```python
from build123d import *

# Parameters (mm, degrees)
SKETCH1_R = 20
SKETCH2_R = 16
SKETCH3_R = 17
SKETCH4_R = 10


with BuildPart() as part:
    # Sketch1 → Loft1 section 0
    with BuildSketch(Plane.XY):
        Circle(SKETCH1_R)
    # Sketch2 → Loft1 section 1
    with BuildSketch(Plane.XY.offset(100)):
        Circle(SKETCH2_R)
    loft()

    # Sketch3 → section 1 of loft4
    with BuildSketch(Plane.XY.offset(200), mode=Mode.PRIVATE) as loft4_s1:
        Circle(SKETCH3_R)
    # loft up to a face of the part (loft4)
    loft([Face(Wire([part.edges().sort_by_distance((-10.952753695, 11.663498039, 100))[0]])), loft4_s1.sketch])

    # Sketch4 → section 1 of loft5
    with BuildSketch(Plane.XY.offset(300), mode=Mode.PRIVATE) as loft5_s1:
        Circle(SKETCH4_R)
    # loft up to a face of the part (loft5)
    loft([Face(Wire([part.edges().sort_by_distance((-11.637300801, 12.392466666, 200))[0]])), loft5_s1.sketch])


solid = part.part
```
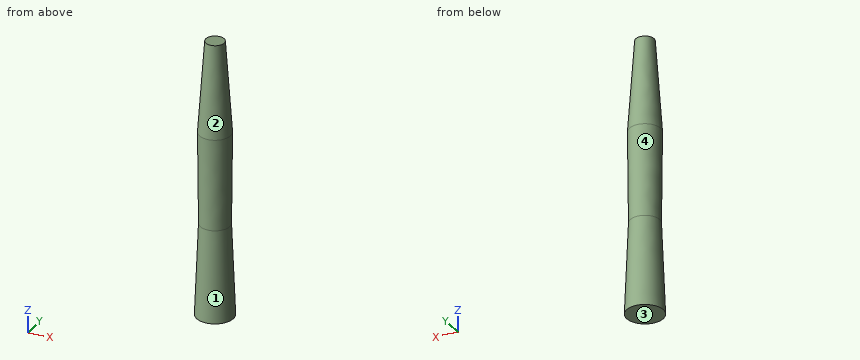
Read the model definition and answer for the solid it produces. Units are mm, in the model's axes. Face numbers are marked on the shaded views. Give positions to 0.01 mm unless a question says otherwise; leave off trailing zeros. Order: outer loops, then holes, each group sorted by start corner. A loop starts at its lowest first (then second) coordinate and runs counter-clockwise, first axis right, second up. Notation, with made-up numbers: (65, 36.25) -> (82, 36.25) arc R21 ccw to (82, 49.25) -> close; hole circle Ø10 at (25, 14.5). An arc over 180 degrees is marked (long way). Write item = value, one per line.
1. Given pin 1 (10 mm diameter, centred on y = -2, z = 189.5, fed in from -X); pin 2 (10 mm diameter, centred on x = 11, y = -15.5, fed in from -Z); pin 3 (8 mm diameter, centred on x = 15.5, z = 36.5, fed in from -Y); pin 4 (2 mm diameter, centred on y = 15, z = 246, fed in from +X) (3 decimals), each flat-ended and moving along its own axis, determine where each tip first touches the part or whether it passes through.
Numbers:
pin_1 = -16.94
pin_2 = 0
pin_3 = -14.55
pin_4 = through
2. A cutting plane is placed at B-B, the plane z = 205. Write down the section's boundary in (x, y), and give its area (3 significant figures).
Numbers:
outline = circle Ø33.3 at (0, 0)
area = 871 mm²
3. The mould has two halves that part along Z. Classify the marked faces 1, 2, 3 and 4: +Z half, -Z half, draft (parallel to the pull), parting line (faces both ways), or undercut.
Numbers:
face_1 = undercut
face_2 = +Z half
face_3 = -Z half
face_4 = undercut
4. A cutting plane is placed at A-A, the plane z = 26. Write down the section's boundary in (x, y), and give its area (3 significant figures).
Numbers:
outline = circle Ø37.92 at (0, 0)
area = 1,130 mm²
5. Straight lines are drawn through the part: line 1 along Y through (x, z) = (-1, 75); line 2 along X through (y, z) = (2, 141.5); line 3 along Y through (x, z) = (12, 252). For each, find the intervals that lie inside material, in ascending order.
Numbers:
line_1 = -16.97 to 16.97
line_2 = -16.29 to 16.29
line_3 = -5.87 to 5.87
